Could you check a few things on this model? Use its own coordinates, in mm. A direction names the side the tool comes from. Give positions to 0.01 mm unless a question says otherwise; leave off trailing zeros. Order: outer loops, then holes, each group sorted by start corner. A loop starts at its lowest first (then second) coordinate and runs counter-clockwise, first axis right, second up. Notation, with made-up numbers: (12, 24.5) -> (41, 24.5) arc R36 cw to (41, 61.5) -> close; hole circle Ø7 at (-9.5, 8). An arc over 180 degrees is marked (long way). One line per item, written item: value.
```python
from build123d import *

# Parameters (mm, degrees)
SKETCH1_W                 = 67.008250425
SKETCH1_H                 = 70
BOSS_EXTRUDE1_DEPTH       = 1.5
BOSS_EXTRUDE2_START       = -9.75
BOSS_EXTRUDE2_DEPTH       = 70
CUT_EXTRUDE1_START        = -6
CUT_EXTRUDE1_OUTLINE_W    = 73
CUT_EXTRUDE1_OUTLINE_H    = 4
CUT_EXTRUDE1_DEPTH        = 1.741494861
SKETCH4_W                 = 8
SKETCH4_H                 = 4.5
SKETCH4_W_2               = 5
SKETCH4_H_2               = 1.5
BOSS_EXTRUDE3_DEPTH       = 3
MIRROR2_COPY_1_SKETCH_W   = 8
MIRROR2_COPY_1_SKETCH_H   = 4.5
MIRROR2_COPY_1_SKETCH_W_2 = 5
MIRROR2_COPY_1_SKETCH_H_2 = 1.5
MIRROR2_COPY_1_DEPTH      = 3
CUT_EXTRUDE2_DEPTH        = 0.5


with BuildPart() as part:
    # Sketch1 → Boss-Extrude1 (new body)
    with BuildSketch(Plane.XY):
        with Locations((29.175646202, 25.25)):
            Rectangle(SKETCH1_W, SKETCH1_H)
    extrude(amount=BOSS_EXTRUDE1_DEPTH)

    # Boss-Extrude2: read off the stored shape, not the designer's step
    # Boss-Extrude2 outline → Boss-Extrude2 (add)
    with BuildSketch(Plane(origin=(0, 0, 0), x_dir=(1, 0, 0), z_dir=(0, 1, 0)).offset(BOSS_EXTRUDE2_START)):
        Polygon((62.952808957, -1.5), (62.679771414, 0), (62.679771414, -1.5), align=None)
    extrude(amount=BOSS_EXTRUDE2_DEPTH)

    # Cut-Extrude1: read off the stored shape, not the designer's step
    # Cut-Extrude1 outline → Cut-Extrude1 (cut)
    with BuildSketch(Plane(origin=(0, 0, 0), x_dir=(0, 1, 0), z_dir=(0.9838340738940914, 0, -0.17908242528220206)).offset(CUT_EXTRUDE1_START)):
        with Locations((25.5, 0)):
            Rectangle(CUT_EXTRUDE1_OUTLINE_W, CUT_EXTRUDE1_OUTLINE_H)
    extrude(amount=CUT_EXTRUDE1_DEPTH, mode=Mode.SUBTRACT)

    # Sketch4 → Boss-Extrude3 (add)
    with BuildSketch(Plane(origin=(0, 0, 0), x_dir=(-1, 0, 0), z_dir=(0, 0, -1))):
        with Locations((-1.171520989, 56.5)):
            Rectangle(SKETCH4_W, SKETCH4_H)
        with Locations((-1.171520989, 56.5)):
            Rectangle(SKETCH4_W_2, SKETCH4_H_2, mode=Mode.SUBTRACT)
    boss_extrude3 = extrude(amount=BOSS_EXTRUDE3_DEPTH)

    # Mirror1: Boss-Extrude3 across plane
    add(boss_extrude3.mirror(Plane(origin=(29.175646202, 0, 0), x_dir=(0, 0, 1), z_dir=(1, 0, 0))))

    # Mirror2: Boss-Extrude3 across plane
    add(boss_extrude3.mirror(Plane(origin=(0, 25.25, 0), x_dir=(0, 0, 1), z_dir=(0, -1, 0))))

    # Mirror2 copy 1 sketch → Mirror2 copy 1 (add)
    with BuildSketch(Plane(origin=(58.351292403, 50.5, 0), x_dir=(1, 0, 0), z_dir=(0, 0, -1))):
        with Locations((-1.171520989, 56.5)):
            Rectangle(MIRROR2_COPY_1_SKETCH_W, MIRROR2_COPY_1_SKETCH_H)
        with Locations((-1.171520989, 56.5)):
            Rectangle(MIRROR2_COPY_1_SKETCH_W_2, MIRROR2_COPY_1_SKETCH_H_2, mode=Mode.SUBTRACT)
    extrude(amount=MIRROR2_COPY_1_DEPTH)

    # Sketch6 → Cut-Extrude2 (cut)
    with BuildSketch(Plane.XY.offset(1.5)):
        Polygon((45.526638666, 38.865120313), (49.152363366, 52.505438829), (1.944558532, 25.25), (49.152363366, -2.005438829), (45.526638666, 11.634879687), (21.944558532, 25.25), align=None)
    extrude(amount=-CUT_EXTRUDE2_DEPTH, mode=Mode.SUBTRACT)


solid = part.part
```
1) Suppose I cut it at D-D, the plane x = 52. Write out the boundary of the cut face in (y, z).
Answer below:
outline: (-9.75, 0) -> (60.25, 0) -> (60.25, 1.5) -> (-9.75, 1.5) -> close
2) If I drill on line 1 along Y through (x, z) = (2, -1.5); line 2 along Z through (x, y) = (16, 20); line 3 along Z through (x, y) = (52, 43.5), over which ranges is the centre line in solid material (lowest first)?
Answer below:
line 1: y = -8.25 to -6.75, -5.25 to -3.75, 54.25 to 55.75, 57.25 to 58.75
line 2: z = 0 to 1
line 3: z = 0 to 1.5
3) Suppose I cut it at C-C, the plane x = 14.5. Write out the boundary of the cut face in (y, z).
Answer below:
outline: (-9.75, 0) -> (60.25, 0) -> (60.25, 1.5) -> (32.5, 1.5) -> (32.5, 1) -> (18, 1) -> (18, 1.5) -> (-9.75, 1.5) -> close
4) For P1, Ø3, axis at x = 48, y = 42, coming from the -Z side; P2, Ø1.2, axis at y = -6, z = -2, coming from the -X side; P3, Ø2.5, axis at x = 59, z = -2, coming from the -Y side, each with a flat end and sliding along its axis, tell me the tip position at first contact or that it passes through.
Answer below:
P1: stops at z = 0
P2: stops at x = -2.83
P3: stops at y = -8.25
5) We'd pull the mould along X, two halves only. Please class faces 5 (the flat face through (57, -3.75, -1)), 6 (the flat face through (61.18, 56, -1)), 7 (the flat face through (3.672, 56, -1)): +X half, -X half, draft (parallel to the pull), parting line (faces both ways), or undercut.
Answer below:
face 5: draft
face 6: +X half
face 7: undercut
6) Suppose I cut it at A-A, the plane z = -2.2. State how many separate pieces and enclosed holes the cut face has, then the cut area to 3 significant figures.
Answer below:
separate pieces: 4
enclosed holes: 4
area: 114 mm2
7) Suppose I cut it at B-B, the plane y = 41. Write out the boundary of the cut face in (x, z).
Answer below:
outline: (-4.33, 0) -> (62.68, 0) -> (62.95, 1.5) -> (46.09, 1.5) -> (46.09, 1) -> (29.22, 1) -> (29.22, 1.5) -> (-4.06, 1.5) -> close
8) For faces 1 (the flat face through (1, -3.75, -1)), 2 (the flat face through (57, -6, 0)), 3 (the flat face through (61.18, -6, -1)), 4 (the flat face through (33.901, 18.347, 1.254)), which set-ups out of +Z, -Z, +X, -X, +Y, -Y let a thin tool reach every point of the face, with its end or its side?
Answer below:
face 1: -Z, +X, -X
face 2: -Z
face 3: -Z, +X, +Y, -Y
face 4: +Z
